Here's how the part is built. I have some questions about the finished solid (model axes, mm). A direction names the side the tool comes from. Coordinates: 2 decimals unless noted, no trailing zeros. Loops run counter-clockwise (first coordinate to the right, second up) from the corner with the lowest first, then second, coordinate; pieces in that order, holes last. Notation, with made-up numbers: (83.25, 31.25) -> (126.25, 31.25) arc R30 ccw to (126.25, 69.25) -> close; hole circle Ø7 at (-39.75, 30.25). An arc over 180 degrees is marked (long way). Answer as a JSON object with one key per item and string values. Group by question number.
1) Which directions (+Z, -Z, +X, -X, +Y, -Y) give clear straight access to the entire face, cutting with the end or side of a thin tool? Please do faces 1 (the cylindrical face through (-8.43, -11.4, 5.54)), 2 (the cylindrical face through (8.43, -11.4, 23.46)), 3 (the flat face through (7.755, -10.368, 5.916)), 4 (the flat face through (0, -12, 24)), 5 (the flat face through (0, -15, 14)).
2) I want a section at C-C (x = 3). Write out the boundary of the cut face in (y, z) (3 decimals).
3) I want a section at B-B (y = -13.25). Write out the boundary of the cut face in (x, z), then the cut area to 3 significant figures.
4) I want a section at A-A (z = 6.5). Write out the boundary of the cut face in (x, y), then the cut area to 3 significant figures.
5) I need wall thicknesses on probe 1 along Z at (x, y) = (-2.5, -12.5); probe 2 along Z at (x, y) = (-6.75, -3.5); probe 3 along X at (y, z) = (-10.5, 15.75). Which ranges of each line are inside material? Lowest first, please. Write a range as [from, to].
6) I want a section at D-D (z = 22.5). Write out the boundary of the cut face in (x, y) (3 decimals).
7) I'm going to push flat-ended pins straight in: pin 1 (2.5 mm diameter, centred on x = -3, z = 23.5, fed in from +Y); pin 2 (6 mm diameter, centred on x = 2.5, z = 8.5, fed in from +Y); pin 3 (1 mm diameter, centred on x = -2, y = -11, fed in from -Z); pin 4 (4 mm diameter, centred on y = -6, z = 5, fed in from +X). Where does each tip first touch, or does it pass through?
8) If we mould it in two halves opening along Z, with no side actions, what happens to faces 6 (the flat face through (9, -9, 20)), 7 (the flat face through (0, -9, 28)), 8 (the flat face through (0, -13, 3))? For each: +Z half, -Z half, draft (parallel to the pull), parting line (faces both ways), or undercut.
Autodesk Fusion 360 part; units mm, degrees
sketch "Sketch1" plane through (0, 0, 0) normal (0, 0, 1) x (1, 0, 0)
  circle A0 centre (0, 0) radius 11.45
  line L0 (-6.8705, 11.9) -> (-13.7409, 0)
  line L1 (-13.7409, 0) -> (-6.8705, -11.9)
  line L2 (-6.8705, -11.9) -> (6.8705, -11.9)
  line L3 (6.8705, -11.9) -> (13.7409, 0)
  line L4 (13.7409, 0) -> (6.8705, 11.9)
  line L5 (6.8705, 11.9) -> (-6.8705, 11.9)
  line L6 (-4.6188, 8) -> (-9.2376, 0)
  line L7 (-9.2376, 0) -> (-4.6188, -8)
  line L8 (-4.6188, -8) -> (4.6188, -8)
  line L9 (4.6188, -8) -> (9.2376, 0)
  line L10 (9.2376, 0) -> (4.6188, 8)
  line L11 (4.6188, 8) -> (-4.6188, 8)
  circle A1 centre (0, 0) radius 6.375
  dimension "d2" = 22.9
  dimension "d3" = 11.9
  dimension "d15" = 8
  dimension "d24" = 12.75
extrude "Extrude2" add sketch "Sketch1" along normal blind 12 contours A0 | L0 L1 L2 L3 L4 L5 | L6 L7 L8 L9 L10 L11 | A1 makes body 1
extrude "Extrude3" add sketch "Sketch1" along normal blind 6.5 from surface at 12 contours A0 | L6 L7 L8 L9 L10 L11 | A1 bodies 1
extrude "Extrude4" add sketch "Sketch1" along normal blind 10 from surface at 18.5 contours A1 bodies 1
sketch "Sketch2" plane through (0, 0, 0) normal (0, 1, 0) x (1, 0, 0)
  line L0 (-9, 0) -> (9, 0)
  line L1 (9, 0) -> (9, -28)
  line L2 (9, -28) -> (-9, -28)
  line L3 (-9, -28) -> (-9, 0)
  dimension "d25" = 28
extrude "Extrude5" add sketch "Sketch2" against normal blind 15 separate body makes body 2
combine "Combine1" operation cut target body 2 tool bodies 1 keep tools
sketch "Sketch3" plane through (9, 0, 0) normal (1, 0, 0) x (0, 1, 0)
  line L0 (0, 28) -> (-15, 28)
  line L1 (-15, 28) -> (-15, 0)
  line L2 (-15, 0) -> (-8.2115, 0)
  line L3 (-14, 26) -> (-12, 26)
  line L4 (-12, 26) -> (-12, 21)
  line L5 (-12, 21) -> (-14, 21)
  line L6 (-14, 21) -> (-14, 26)
  line L7 (-14, 3) -> (-12, 3)
  line L8 (-12, 3) -> (-12, 8)
  line L9 (-12, 8) -> (-14, 8)
  line L10 (-14, 8) -> (-14, 3)
  line L11 (-7.0783, 12) -> (-7.0783, 18.5)
  line L12 (-8.2115, 0) -> (-8.2115, 12)
  line L13 (-8.2115, 12) -> (-7.0783, 12)
  line L14 (-7.0783, 18.5) -> (0, 18.5)
  line L15 (0, 18.5) -> (0, 28)
  dimension "d28" = 2
  dimension "d29" = 5
  dimension "d30" = 2
  dimension "d31" = 5
  dimension "d32" = 3
  dimension "d33" = 2
extrude "Extrude6" cut sketch "Sketch3" against normal blind 28 contours L3 L4 L5 L6 | L7 L8 L9 L10 bodies 2
fillet "Fillet1" radius 2 4 edges at (9, -12, 23.5) (9, -12, 5.5) (-9, -12, 23.5) (-9, -12, 5.5) on bodies 2
fillet "Fillet2" radius 1 8 edges at (-9, -7.0783, 15.25) (-9, -8.2115, 6) (9, -8.2115, 6) (9, -7.0783, 15.25) (-6.375, 0, 23.25) (-9, 0, 23.25) (6.375, 0, 23.25) (9, 0, 23.25) on bodies 2
hidden bodies 1
equation "d3 = 23.8 mm / 2"
equation "d9 = 18.5 mm - 12 mm"
equation "d30 = d28"
equation "d31 = d29"
equation "d33 = d28"
Determined:
{
 "1": {"face 1": "-X", "face 2": "+X", "face 3": "-Z, +Y", "face 4": "+X, -X", "face 5": "+Z, -Z, +X, -X, -Y"},
 "2": {"outline": "(-15, 0) -> (-11.9, 0) -> (-11.9, 12) -> (-11.05, 12) -> (-11.05, 18.5) -> (-5.625, 18.5) -> (-5.625, 28) -> (-15, 28) -> close; hole (-14, 3) -> (-12, 3) -> (-12, 8) -> (-14, 8) -> close; hole (-14, 21) -> (-12, 21) -> (-12, 26) -> (-14, 26) -> close"},
 "3": {"outline": "(-9, 0) -> (9, 0) -> (9, 3) -> (-9, 3) -> close; (-9, 8) -> (9, 8) -> (9, 21) -> (-9, 21) -> close; (-9, 26) -> (9, 26) -> (9, 28) -> (-9, 28) -> close", "area": "324 mm^2"},
 "4": {"outline": "(-9, -15) -> (9, -15) -> (9, -14) -> (-9, -14) -> close; (-9, -10) arc R2 ccw to (-7, -12) -> (7, -12) arc R2 ccw to (9, -10) -> (9, -9.54) arc R1 ccw to (8.66, -8.79) -> (6.87, -11.9) -> (-6.87, -11.9) -> (-8.66, -8.79) arc R1 ccw to (-9, -9.54) -> close", "area": "25.6 mm^2"},
 "5": {"probe 1": "[0, 3], [8, 21], [26, 28]", "probe 2": "[18.5, 28]", "probe 3": "[-9, -4.57], [4.57, 9]"},
 "6": {"outline": "(-9, -15) -> (9, -15) -> (9, -14) -> (-9, -14) -> close; (-9, -10) arc R2 ccw to (-7, -12) -> (7, -12) arc R2 ccw to (9, -10) -> (9, -1) arc R1 ccw to (8, 0) -> (7.307, 0) arc R1 ccw to (6.316, -0.864) arc R6.375 cw to (-6.316, -0.864) arc R1 ccw to (-7.307, 0) -> (-8, 0) arc R1 ccw to (-9, -1) -> close"},
 "7": {"pin 1": "y = -4.75", "pin 2": "y = -11.9", "pin 3": "z = 12", "pin 4": "through"},
 "8": {"face 6": "draft", "face 7": "+Z half", "face 8": "undercut"}
}
